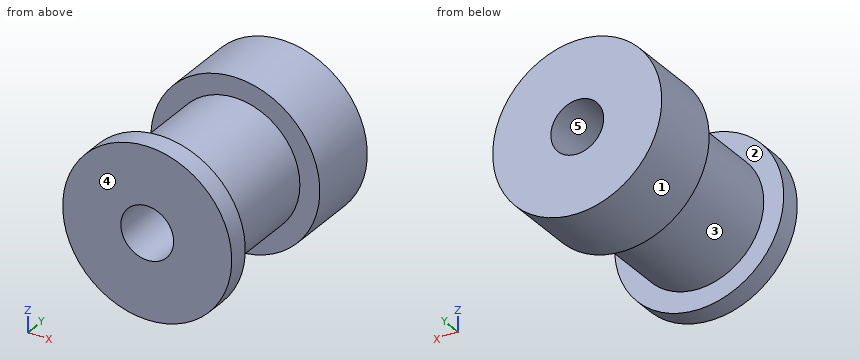
from build123d import *

# Parameters (mm, degrees)
SKETCH_1_R          = 8
EXTRUDE_1_DEPTH     = 7
SKETCH_2_R          = 6.11
EXTRUDE_2_DEPTH     = 11
EXTRUDE_START       = 2
SKETCH_3_R          = 8
EXTRUDE_3_DEPTH     = 2
SKETCH_4_R          = 2.5
CUT_EXTRUDE_1_DEPTH = 25


with BuildPart() as part:
    # 草图1 → 凸台-拉伸1 (new body)
    with BuildSketch(Plane(origin=(0, 0, 0), x_dir=(1, 0, 0), z_dir=(0, 1, 0))):
        with Locations(Location((0, 0, 0), (0, 0, 270))):
            Circle(SKETCH_1_R)
    extrude(amount=EXTRUDE_1_DEPTH)

    # 草图2 → 凸台-拉伸2 (add)
    with BuildSketch(Plane.XZ):
        with Locations(Location((0, 0, 0), (0, 0, 270))):
            Circle(SKETCH_2_R)
    extrude(amount=EXTRUDE_2_DEPTH)

    # 草图3 → 凸台-拉伸3 (add)
    with BuildSketch(Plane.XZ.offset(11).offset(EXTRUDE_START)):
        with Locations(Location((0, 0, 0), (0, 0, 90))):
            Circle(SKETCH_3_R)
    extrude(amount=-EXTRUDE_3_DEPTH)

    # 草图4 → 切除-拉伸1 (cut)
    with BuildSketch(Plane(origin=(0, 7, 0), x_dir=(1, 0, 0), z_dir=(0, 1, 0))):
        with Locations(Location((0, 0, 0), (0, 0, 270))):
            Circle(SKETCH_4_R)
    extrude(amount=-CUT_EXTRUDE_1_DEPTH, mode=Mode.SUBTRACT)


solid = part.part
Can you work these out from the model? Positions are in its coordinate system, mm. Face numbers are marked on the shaded views. A direction names the side the tool comes from. Round coordinates to 2 decimals unless told otherwise and drop trailing zeros. Order: outer loops, then holes, each group sorted by start corner. A loop starts at its lowest first (then second) coordinate and runs counter-clockwise, first axis right, second up. Notation, with made-up numbers: M 77.5,32 L 81.5,32 A11 cw 81.5,40 Z; hole C 83.25,8 d2. An arc over 180 degrees is marked long. Use a Markdown table: item, result.
1) If we mould it in two halves opening along X, with no side actions, what happens to the marked faces 3, 4 and 5? For each: +X half, -X half, draft (parallel to the pull), parting line (faces both ways), or undercut.
Geometry says:
| item | result |
|---|---|
| face 3 | parting line |
| face 4 | draft |
| face 5 | undercut |
2) I'm going to push flat-ended pins straight in: P1, Ø1, axis at y = 0, z = 2.5, coming from the +X side; P2, Ø1, axis at y = -6.5, z = -4.5, coming from the -X side; P3, Ø2, axis at x = -1.5, y = 1.5, coming from the -Z side; P4, Ø4.5, axis at x = 0, z = 0, coming from the -Y side. Where does each tip first touch, or does it pass through?
Geometry says:
| item | result |
|---|---|
| P1 | stops at x = 7.75 |
| P2 | stops at x = -4.62 |
| P3 | stops at z = -7.98 |
| P4 | passes through |
3) If I drill on line 1 along Y through (x, z) = (-4, -4.75); line 2 along X through (y, z) = (-0.5, 0); line 3 along X through (y, z) = (0.25, 0), over which ranges is the centre line in solid material (lowest first)?
Geometry says:
| item | result |
|---|---|
| line 1 | y = -13 to -11, 0 to 7 |
| line 2 | x = -6.11 to -2.5, 2.5 to 6.11 |
| line 3 | x = -8 to -2.5, 2.5 to 8 |
4) Imagine slicing it at A-A (x = 0). List the corners of the cut face in (y, z) for me.
Geometry says:
| item | result |
|---|---|
| outline | M -13,-8 L -11,-8 L -11,-6.11 L 0,-6.11 L 0,-8 L 7,-8 L 7,-2.5 L -13,-2.5 Z; M -13,2.5 L 7,2.5 L 7,8 L 0,8 L 0,6.11 L -11,6.11 L -11,8 L -13,8 Z |
5) On a 3-axis mill with a long thin cutter (end or side, diameter ignored), from which of +Z, -Z, +X, -X, +Y, -Y can I reach the whole of each face in a straight line? I mean the marked faces 1 and 2. Say none if no direction works.
Geometry says:
| item | result |
|---|---|
| face 1 | +Y, -Y |
| face 2 | none |
6) Imagine slicing it at D-D (x = -5). List the corners of the cut face in (y, z) for me (3 decimals).
Geometry says:
| item | result |
|---|---|
| outline | M -13,-6.245 L -11,-6.245 L -11,-3.512 L 0,-3.512 L 0,-6.245 L 7,-6.245 L 7,6.245 L 0,6.245 L 0,3.512 L -11,3.512 L -11,6.245 L -13,6.245 Z |
7) Imagine slicing it at C-C (y = -6.75). List the corners of the cut face in (x, z) for me.
Geometry says:
| item | result |
|---|---|
| outline | C 0,0 d12.22; hole C 0,0 d5 |
8) Imagine slicing it at B-B (z = 0). List the corners of the cut face in (x, y) for me, then the cut area to 3 significant figures.
Geometry says:
| item | result |
|---|---|
| outline | M -8,-13 L -2.5,-13 L -2.5,7 L -8,7 L -8,0 L -6.11,0 L -6.11,-11 L -8,-11 Z; M 2.5,-13 L 8,-13 L 8,-11 L 6.11,-11 L 6.11,0 L 8,0 L 8,7 L 2.5,7 Z |
| area | 178 mm² |
